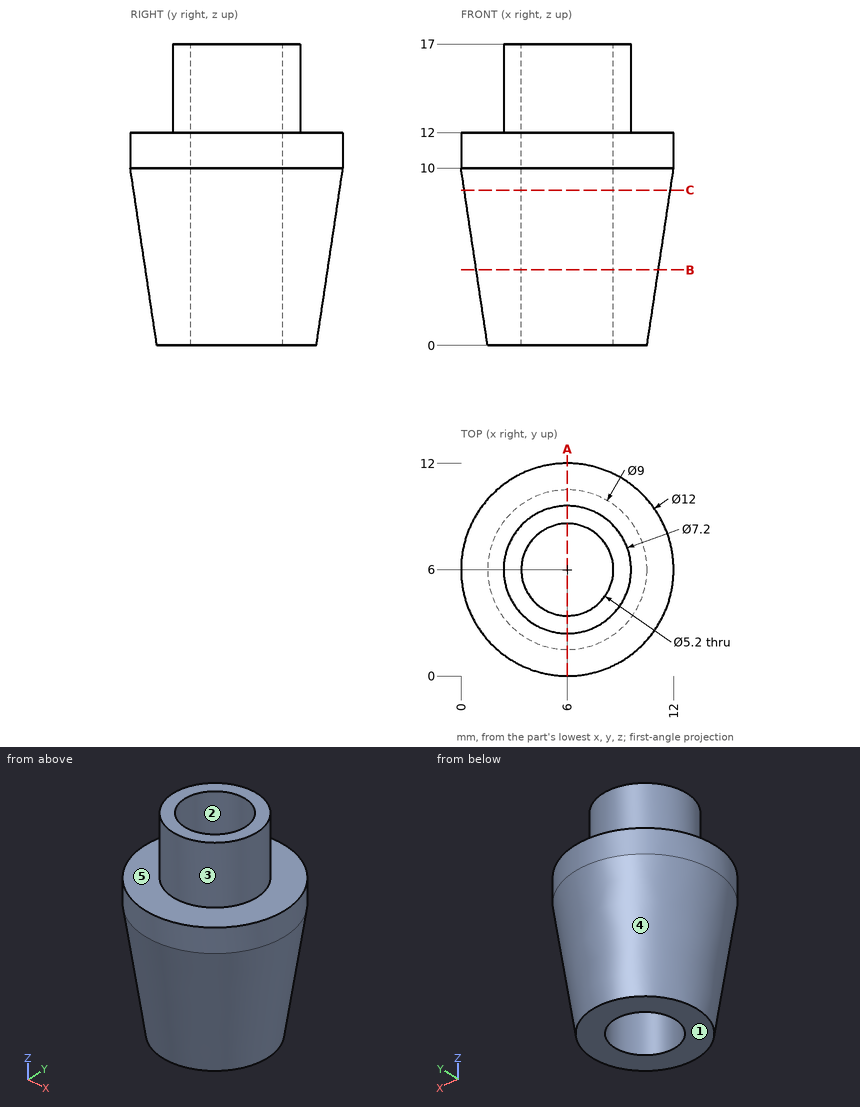
The figure shows three views and two pictorial views of one solid part (mm, origin at its lowest corner). Answer the questions. A direction names the side the tool comes from. Round coordinates to 2 decimals unless told otherwise and drop trailing zeros. Loops run counter-clockwise (first coordinate to the right, second up) from the corner with the lowest first, then second, coordinate; pieces in that order, holes last. Notation, with made-up numbers: M 65.25,73.5 L 80.25,73.5 A21 ccw 80.25,103.5 Z; hole C 11.25,52 d7. An arc over 180 degrees is marked long. Write each question's results on one line, items separated by ' | '. Start each with the question number.
1) Which of the six approach directions +Z, -Z, +X, -X, +Y, -Y give full straight-line access (tool end or side, diameter ignored) to the marked faces 4 and 5?
2) Determine the mould class of the marked faces 1, 2 and 3 for opening direction Y: pulls with the +Y half, pulls with the -Y half, needs draft (parallel to the pull), parting line crosses it, or undercut.
3) Straight lines are drawn through the part: probe 1 along Y at (x, z) = (6, 13); probe 2 along Y at (x, z) = (6, 9); probe 3 along X at (y, z) = (8.25, 14.25). For each, find the intervals that lie inside material, in ascending order.
4) Each of these flat-tipped pins is pushed along its axis until it touches: pin 1 (4 mm diameter, centred on y = 8, z = 5, fed in from -X); pin 2 (1.5 mm diameter, centred on x = 4.5, y = 7, fed in from -Z). Where does it stop, or does it pass through?
5) Find section A-A on x = 6. Write down the section's boundary in (y, z), plus the area to 3 significant figures.
6) Find section B-B on z = 4.25. Write down the section's boundary in (x, y) (1 decimal), plus the area to 3 significant figures.
7) Find section C-C on z = 8.75. Write down the section's boundary in (x, y) (1 decimal), plus the area to 3 significant figures.
Final values:
1) face 4: -Z | face 5: +Z
2) face 1: needs draft | face 2: undercut | face 3: parting line crosses it
3) probe 1: 2.4 to 3.4, 8.6 to 9.6 | probe 2: 0.15 to 3.4, 8.6 to 11.85 | probe 3: 3.19 to 4.7, 7.3 to 8.81
4) pin 1: x = 0.57 | pin 2: through
5) outline: M 0,10 L 1.5,0 L 3.4,0 L 3.4,17 L 2.4,17 L 2.4,12 L 0,12 Z; M 8.6,0 L 10.5,0 L 12,10 L 12,12 L 9.6,12 L 9.6,17 L 8.6,17 Z | area: 76.6 mm²
6) outline: C 6,6 d10.3; hole C 6,6 d5.2 | area: 61.7 mm²
7) outline: C 6,6 d11.6; hole C 6,6 d5.2 | area: 84.9 mm²
